Could you check a few things on this model? Use its own coordinates, in mm. Face numbers are marked on the shaded views. A direction names the side the tool comes from. Round coordinates to 2 decimals unless told otherwise and drop trailing zeros. Loops run counter-clockwise (first coordinate to the right, second up) from the corner with the lowest first, then second, coordinate; pieces in that order, holes last. Notation, with made-up numbers: (54, 89) -> (61, 89) arc R28 ccw to (61, 127) -> close; hole circle Ø2 at (47.25, -36.75). An arc over 180 degrees is marked (long way). Put each result on its own line as item: value. Start each with the question number.
1. Imagine slicing it at D-D, the plane z = 7. Please give me the cut outline in (x, y), and give its area (3 significant figures).
2. I need wall thicknesses on line 1 (X direction, y = 0.55, z = 11.5) (3 decimals); line 2 (Y direction, x = 3, z = -7); line 3 (X direction, y = -3.25, z = -12.5). Which ranges of each line are inside material? Lowest first, please. Write a range as [from, to].
3. Imagine slicing it at C-C, the plane y = 3.5. Please give me the cut outline in (x, z) (3 decimals), and give its area (3 significant figures).
4. Imagine slicing it at A-A, the plane z = -5. Please give me the cut outline in (x, y).
5. Imagine slicing it at B-B, the plane x = 27. Please give me the cut outline in (y, z), and give its area (3 significant figures).
6. I'm going to push flat-ended pins straight in: P1, Ø1, axis at x = -19.5, y = 2, coming from the -Z side; P2, Ø1.2, axis at y = 2, z = 1, coming from the +X side; P3, Ø3.5, axis at x = -29, z = 11.5, coming from the +Y side; P4, Ø10, axis at y = 2.5, z = -1, coming from the -X side. Where does each tip first touch, or does it pass through?
7. Which directions (+Z, -Z, +X, -X, +Y, -Y) give clear straight access to the entire face, cutting with the end or side of a thin tool? Please do the marked faces 1, 2, 3 and 4.
```python
from build123d import *

# Parameters (mm, degrees)
EXTRUDE_1_DEPTH     = 1.2
SKETCH_2_R          = 1.375
CUT_EXTRUDE_1_DEPTH = 1.2
SKETCH_11_W         = 51.4
SKETCH_11_H         = 5.1
EXTRUDE_9_DEPTH     = 8.6
SKETCH_12_W         = 6.45
SKETCH_12_H         = 6.45
EXTRUDE_10_DEPTH    = 1.5
SKETCH_13_R         = 3.1
EXTRUDE_11_DEPTH    = 11.2
SKETCH_14_W         = 28.31
SKETCH_14_H         = 27.71
EXTRUDE_12_DEPTH    = 5
SKETCH_15_W         = 26.63
SKETCH_15_H         = 14.03
EXTRUDE_13_DEPTH    = 0.28
SKETCH_16_W         = 3.87
SKETCH_16_H         = 9.47
EXTRUDE_14_DEPTH    = 0.1
SKETCH_17_W         = 28.31
SKETCH_17_H         = 3.337027264
CUT_EXTRUDE_2_DEPTH = 25


with BuildPart() as part:
    # 草图1 → 凸台-拉伸1 (new body)
    with BuildSketch(Plane(origin=(0, 0, 0), x_dir=(1, 0, 0), z_dir=(0, 1, 0))):
        with BuildLine():
            Line((-29.5, 15), (29.5, 15))
            ThreePointArc((29.5, 15), (31.621320344, 14.121320344), (32.5, 12))
            Line((32.5, 12), (32.5, -12))
            ThreePointArc((32.5, -12), (31.621320344, -14.121320344), (29.5, -15))
            Line((29.5, -15), (-29.5, -15))
            ThreePointArc((-29.5, -15), (-31.621320344, -14.121320344), (-32.5, -12))
            Line((-32.5, -12), (-32.5, 12))
            ThreePointArc((-32.5, 12), (-31.621320344, 14.121320344), (-29.5, 15))
        make_face()
    extrude(amount=EXTRUDE_1_DEPTH)

    # 草图2 → 切除-拉伸1 (cut)
    with BuildSketch(Plane(origin=(0, 1.2, 0), x_dir=(1, 0, 0), z_dir=(0, 1, 0))):
        with Locations(Location((29, -11.5, 0), (0, 0, 270))):
            Circle(SKETCH_2_R)
        with Locations(Location((29, 11.5, 0), (0, 0, 270))):
            Circle(SKETCH_2_R)
        with Locations(Location((-29, -11.5, 0), (0, 0, 270))):
            Circle(SKETCH_2_R)
        with Locations(Location((-29, 11.5, 0), (0, 0, 270))):
            Circle(SKETCH_2_R)
    extrude(amount=-CUT_EXTRUDE_1_DEPTH, mode=Mode.SUBTRACT)

    # 草图11 → 凸台-拉伸9 (add)
    with BuildSketch(Plane.XZ):
        with Locations((-0.05, -11.55)):
            Rectangle(SKETCH_11_W, SKETCH_11_H)
    extrude(amount=EXTRUDE_9_DEPTH)

    # 草图12 → 凸台-拉伸10 (add)
    with BuildSketch(Plane(origin=(0, 1.2, 0), x_dir=(1, 0, 0), z_dir=(0, 1, 0))):
        with Locations((-27.475, -1.135)):
            Rectangle(SKETCH_12_W, SKETCH_12_H)
    extrude(amount=EXTRUDE_10_DEPTH)

    # 草图13 → 凸台-拉伸11 (add)
    with BuildSketch(Plane(origin=(0, 2.7, 0), x_dir=(1, 0, 0), z_dir=(0, 1, 0))):
        with Locations(Location((-27.475, -1.135, 0), (0, 0, 270))):
            Circle(SKETCH_13_R)
    extrude(amount=EXTRUDE_11_DEPTH)

    # 草图14 → 凸台-拉伸12 (add)
    with BuildSketch(Plane(origin=(0, 1.2, 0), x_dir=(1, 0, 0), z_dir=(0, 1, 0))):
        with Locations((-7.605, 0.645)):
            Rectangle(SKETCH_14_W, SKETCH_14_H)
    extrude(amount=EXTRUDE_12_DEPTH)

    # 草图15 → 凸台-拉伸13 (add)
    with BuildSketch(Plane(origin=(0, 6.2, 0), x_dir=(1, 0, 0), z_dir=(0, 1, 0))):
        with Locations((-7.585, 3.455)):
            Rectangle(SKETCH_15_W, SKETCH_15_H)
    extrude(amount=EXTRUDE_13_DEPTH)

    # 草图16 → 凸台-拉伸14 (add)
    with BuildSketch(Plane(origin=(0, 1.2, 0), x_dir=(1, 0, 0), z_dir=(0, 1, 0))):
        with Locations((27.105, 3.845)):
            Rectangle(SKETCH_16_W, SKETCH_16_H)
    extrude(amount=EXTRUDE_14_DEPTH)

    # 草图17 → 切除-拉伸2 (cut)
    with BuildSketch(Plane.XY.offset(13.21)):
        with Locations((-7.605, 2.868513632)):
            Rectangle(SKETCH_17_W, SKETCH_17_H)
    extrude(amount=-CUT_EXTRUDE_2_DEPTH, mode=Mode.SUBTRACT)


solid = part.part
```
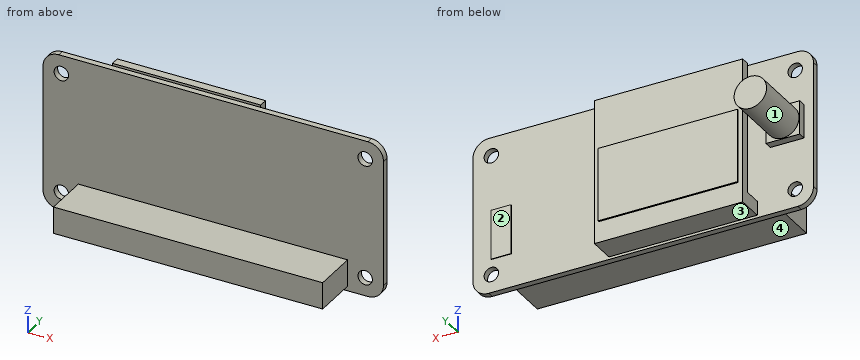
Entries:
1. outline: (-32.5, 0) -> (32.5, 0) -> (32.5, 1.2) -> (-32.5, 1.2) -> close; (-21.76, 4.54) -> (6.55, 4.54) -> (6.55, 6.2) -> (-21.76, 6.2) -> close
1. area: 125 mm^2
2. line 1: [-32.5, -30.375], [-27.625, 27.625], [30.375, 32.5]
2. line 2: [0, 1.2], [4.54, 6.48]
2. line 3: [-25.75, 25.65]
3. outline: circle Ø6.2 at (-27.475, 1.135); (-21.76, -14.5) -> (6.55, -14.5) -> (6.55, -11.79) -> (-21.76, -11.79) -> close
3. area: 107 mm^2
4. outline: (-32.5, 0) -> (32.5, 0) -> (32.5, 1.2) -> (29.04, 1.2) -> (29.04, 1.3) -> (25.17, 1.3) -> (25.17, 1.2) -> (-32.5, 1.2) -> close; (-21.76, 4.54) -> (6.55, 4.54) -> (6.55, 6.2) -> (5.73, 6.2) -> (5.73, 6.48) -> (-20.9, 6.48) -> (-20.9, 6.2) -> (-21.76, 6.2) -> close
5. outline: (0, -15) -> (1.2, -15) -> (1.2, -8.58) -> (1.3, -8.58) -> (1.3, 0.89) -> (1.2, 0.89) -> (1.2, 15) -> (0, 15) -> close
5. area: 36.9 mm^2
6. P1: z = -14.5
6. P2: x = -24.25
6. P3: y = 1.2
6. P4: x = -32.5
7. face 1: +Y
7. face 2: +Z, -Z, +X, +Y
7. face 3: -Z, +X, -X, +Y
7. face 4: -Z, +X, -X, -Y
